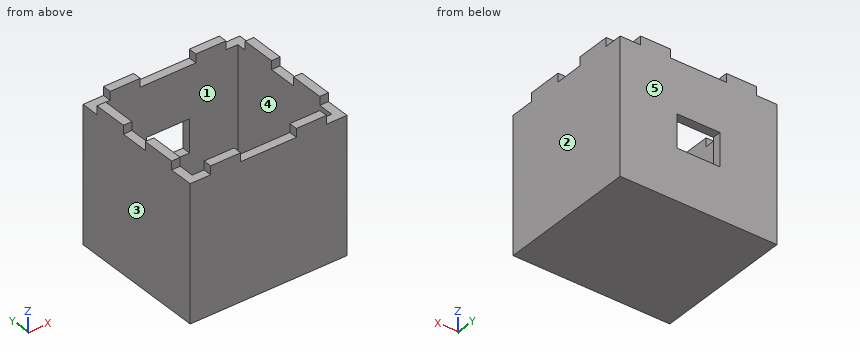
from build123d import *

# Parameters (mm, degrees)
ESBO_O1_W                = 7
ESBO_O1_H                = 2
ESBO_O1_W_2              = 12.960369515
ESBO_O1_W_3              = 2
ESBO_O1_H_2              = 8
ESBO_O1_H_3              = 6.636258661
ESBO_O1_W_4              = 12.96
RESSALTO_EXTRUS_O1_DEPTH = 29.5
ESBO_O1_3_W              = 7
ESBO_O1_3_H              = 2
ESBO_O1_3_W_2            = 2
ESBO_O1_3_H_2            = 8
RESSALTO_EXTRUS_O2_DEPTH = 31.5
ESBO_O1_4_W              = 36.5
ESBO_O1_4_H              = 32.5
RESSALTO_EXTRUS_O3_DEPTH = 2
ESBO_O2_W                = 10
ESBO_O2_H                = 7.7
CORTE_EXTRUS_O1_DEPTH    = 12.596420323


with BuildPart() as part:
    # Esbo_o1 → Ressalto-extrus_o1 (new body)
    with BuildSketch(Plane.XY):
        Polygon((-15.664415021, 7.362009238), (-15.664415021, 9.596420323), (-12.894784536, 9.596420323), (-12.894784536, 11.596420323), (-17.664415021, 11.596420323), (-17.664415021, 7.362009238), align=None)
        with Locations((-9.394784536, 10.596420323)):
            Rectangle(ESBO_O1_W, ESBO_O1_H)
        with Locations((0.585400222, 10.596420323)):
            Rectangle(ESBO_O1_W_2, ESBO_O1_H)
        with Locations((10.565584979, 10.596420323)):
            Rectangle(ESBO_O1_W, ESBO_O1_H)
        Polygon((14.065584979, 11.596420323), (14.065584979, 9.596420323), (16.835584979, 9.596420323), (16.835584979, 7.362009238), (18.835584979, 7.362009238), (18.835584979, 11.596420323), align=None)
        with Locations((17.835584979, 3.362009238)):
            Rectangle(ESBO_O1_W_3, ESBO_O1_H_2)
        with Locations((17.835584979, -3.956120093)):
            Rectangle(ESBO_O1_W_3, ESBO_O1_H_3)
        with Locations((17.835584979, -11.274249423)):
            Rectangle(ESBO_O1_W_3, ESBO_O1_H_2)
        Polygon((18.835584979, -15.274249423), (16.835584979, -15.274249423), (16.835584979, -18.903579677), (14.065584979, -18.903579677), (14.065584979, -20.903579677), (18.835584979, -20.903579677), align=None)
        with Locations((10.565584979, -19.903579677)):
            Rectangle(ESBO_O1_W, ESBO_O1_H)
        with Locations((0.585584979, -19.903579677)):
            Rectangle(ESBO_O1_W_4, ESBO_O1_H)
        with Locations((-9.394415021, -19.903579677)):
            Rectangle(ESBO_O1_W, ESBO_O1_H)
        Polygon((-15.664415021, -18.903579677), (-15.664415021, -15.274249423), (-17.664415021, -15.274249423), (-17.664415021, -20.903579677), (-12.894415021, -20.903579677), (-12.894415021, -18.903579677), align=None)
        with Locations((-16.664415021, -11.274249423)):
            Rectangle(ESBO_O1_W_3, ESBO_O1_H_2)
        with Locations((-16.664415021, -3.956120093)):
            Rectangle(ESBO_O1_W_3, ESBO_O1_H_3)
        with Locations((-16.664415021, 3.362009238)):
            Rectangle(ESBO_O1_W_3, ESBO_O1_H_2)
    extrude(amount=RESSALTO_EXTRUS_O1_DEPTH)

    # Esbo_o1_3 → Ressalto-extrus_o2 (add)
    with BuildSketch(Plane.XY):
        with Locations((-9.394784536, 10.596420323)):
            Rectangle(ESBO_O1_3_W, ESBO_O1_3_H)
        with Locations((10.565584979, 10.596420323)):
            Rectangle(ESBO_O1_3_W, ESBO_O1_3_H)
        with Locations((17.835584979, 3.362009238)):
            Rectangle(ESBO_O1_3_W_2, ESBO_O1_3_H_2)
        with Locations((17.835584979, -11.274249423)):
            Rectangle(ESBO_O1_3_W_2, ESBO_O1_3_H_2)
        with Locations((10.565584979, -19.903579677)):
            Rectangle(ESBO_O1_3_W, ESBO_O1_3_H)
        with Locations((-9.394415021, -19.903579677)):
            Rectangle(ESBO_O1_3_W, ESBO_O1_3_H)
        with Locations((-16.664415021, -11.274249423)):
            Rectangle(ESBO_O1_3_W_2, ESBO_O1_3_H_2)
        with Locations((-16.664415021, 3.362009238)):
            Rectangle(ESBO_O1_3_W_2, ESBO_O1_3_H_2)
    extrude(amount=RESSALTO_EXTRUS_O2_DEPTH)

    # Esbo_o1_4 → Ressalto-extrus_o3 (add)
    with BuildSketch(Plane.XY):
        with Locations((0.585584979, -4.653579677)):
            Rectangle(ESBO_O1_4_W, ESBO_O1_4_H)
    extrude(amount=-RESSALTO_EXTRUS_O3_DEPTH)

    # Esbo_o2 → Corte-extrus_o1 (cut, through all)
    with BuildSketch(Plane(origin=(0, 0, 0), x_dir=(1, 0, 0), z_dir=(0, 1, 0))):
        with Locations((0.585584979, -13.75)):
            Rectangle(ESBO_O2_W, ESBO_O2_H)
    extrude(amount=CORTE_EXTRUS_O1_DEPTH, mode=Mode.SUBTRACT)


solid = part.part
CAD build for the part. Positions are in the model's coordinates, mm. Face numbers are marked on the shaded views. A direction names the side the tool comes from. Give positions to 0.01 mm unless a question says otherwise; leave off trailing zeros. Loops run counter-clockwise (first coordinate to the right, second up) from the corner with the lowest first, then second, coordinate; pieces in that order, holes last. Notation, with made-up numbers: M 85.25,71 L 95.25,71 A17 cw 95.25,78 Z; hole C -37.75,-24 d8. An arc over 180 degrees is marked long. Write each question's results on one line, items separated by ' | '.
Q1. Flat gauge pins, fed straight in: P1, Ø0.6, axis at x = 18, z = 30, coming from the -Y side; P2, Ø1, axis at y = -20, z = 31, coming from the +X side; P3, Ø10, axis at x = 0.5, y = -17, coming from the +Z side. Where does each tip first touch, or does it go through?
Geometry check:
P1: stops at y = -15.27 | P2: stops at x = 14.07 | P3: stops at z = 29.5
Q2. Band-saw the part on B-B on y = -3. Write the cut outline in (x, z).
Geometry check:
outline: M -17.66,-2 L 18.84,-2 L 18.84,29.5 L 16.84,29.5 L 16.84,0 L -15.66,0 L -15.66,29.5 L -17.66,29.5 Z
Q3. Probe probe 1 along X at (y, z) = (-9.5, 4.5); probe 2 along Y at (x, z) = (9, 1.5); probe 3 along Y at (x, z) = (-2.5, 16). List the from-to ranges inside material, lowest first.
Geometry check:
probe 1: x = -17.66 to -15.66, 16.84 to 18.84 | probe 2: y = -20.9 to -18.9, 9.6 to 11.6 | probe 3: y = -20.9 to -18.9
Q4. Which spindle directions (+Z, -Z, +X, -X, +Y, -Y) get a long thin tool onto all of the face, cutting with end or side? Do the marked faces 1 and 2. Say none if no direction does.
Geometry check:
face 1: +Z | face 2: +Z, -Z, +X, +Y, -Y
Q5. Band-saw the part on D-D on x = 16. Write the cut outline in (y, z).
Geometry check:
outline: M -20.9,-2 L 11.6,-2 L 11.6,29.5 L 9.6,29.5 L 9.6,0 L -18.9,0 L -18.9,29.5 L -20.9,29.5 Z
Q6. Band-saw the part on A-A on x = 5. Write the cut outline in (y, z), and give its area (3 significant figures).
Geometry check:
outline: M -20.9,-2 L 11.6,-2 L 11.6,9.9 L 9.6,9.9 L 9.6,0 L -18.9,0 L -18.9,29.5 L -20.9,29.5 Z; M 9.6,17.6 L 11.6,17.6 L 11.6,29.5 L 9.6,29.5 Z | area: 168 mm²
Q7. Mould opens along X. For the marked faces 3, 4 and 5 say: pulls with the +X half, pulls with the -X half, needs draft (parallel to the pull), parting line crosses it, or undercut.
Geometry check:
face 3: pulls with the -X half | face 4: undercut | face 5: needs draft
Q8. Band-saw the part on C-C on z = 2.5. Write the cut outline in (x, y).
Geometry check:
outline: M -17.66,-20.9 L 18.84,-20.9 L 18.84,11.6 L -17.66,11.6 Z; hole M -15.66,-18.9 L 16.84,-18.9 L 16.84,9.6 L -15.66,9.6 Z
